For this review, take the finished solid that the model builds, in its own axes (mm). A direction names the side the tool comes from. Coordinates: 2 decimals unless noted, no trailing zeros. Write each loop counter-clockwise with the first axis right and the second up, starting at its lowest first coordinate (ties: lowest second). Pieces come first, ordered by that corner, then holes. Notation, with made-up numbers: M -36,41.25 L -18,41.25 A20 ccw -18,48.25 Z; hole C 15.5,16.5 d4. An arc over 180 degrees is marked long. Return JSON: item names as keys, results as strings.
```python
from build123d import *

# Parameters (mm, degrees)
F0_R     = 25.4
F1_DEPTH = 228.6
F0_W     = 1422.4
F0_H     = 254
F2_DEPTH = 101.6
F3_DEPTH = 635
F4_W     = 457.2
F4_H     = 177.8
F5_DEPTH = 76.2


with BuildPart() as f1:
    # F0 (on Top) → F1 (new body)
    with BuildSketch(Plane.XY):
        with BuildLine():
            Line((0, 508), (0, 254))
            Line((0, 254), (1422.4, 254))
            Line((1422.4, 254), (1422.4, 508))
            add(Edge.make_bspline(
                [(0, 508), (241.551548, 567.851314), (711.2, 651.348686), (1180.848452, 567.851314), (1422.4, 508)],
                knots=[0, 0, 0, 0, 718.42049, 1436.840979, 1436.840979, 1436.840979, 1436.840979], degree=3))
        make_face()
        with Locations((546.1, 558.8)):
            Circle(F0_R, mode=Mode.SUBTRACT)
        with Locations((876.3, 558.8)):
            Circle(F0_R, mode=Mode.SUBTRACT)
        with Locations((546.1, 558.8)):
            Circle(F0_R)
        with Locations((876.3, 558.8)):
            Circle(F0_R)
    extrude(amount=F1_DEPTH)

    # F0 (on Top) → F2 (join)
    with BuildSketch(Plane.XY):
        with Locations((711.2, 127)):
            Rectangle(F0_W, F0_H)
        with Locations((88.9, 76.2)):
            Circle(F0_R, mode=Mode.SUBTRACT)
        with Locations((1333.5, 76.2)):
            Circle(F0_R, mode=Mode.SUBTRACT)
        with Locations((88.9, 76.2)):
            Circle(F0_R)
        with Locations((1333.5, 76.2)):
            Circle(F0_R)
    extrude(amount=F2_DEPTH)

    # F0 (on Top) → F3 (join)
    with BuildSketch(Plane.XY):
        with Locations((876.3, 558.8)):
            Circle(F0_R)
        with Locations((546.1, 558.8)):
            Circle(F0_R)
        with Locations((1333.5, 76.2)):
            Circle(F0_R)
        with Locations((88.9, 76.2)):
            Circle(F0_R)
    extrude(amount=-F3_DEPTH)

    # F4 (on face) → F5 (join)
    with BuildSketch(Plane(origin=(0, 0, -635), x_dir=(1, 0, 0), z_dir=(0, 0, -1))):
        with Locations((711.2, -520.7)):
            Rectangle(F4_W, F4_H)
    extrude(amount=-F5_DEPTH)


solid = f1.part
```
1. Draft analysis for pull direction X (two halves, no side actions). For faces 4 (the face through (1308.125, 77.317, -313.055)), 5 (the face through (701, 129, 101.6)), 6 (the face through (1422.4, 307, 87)), state which applies: +X half, -X half, draft (parallel to the pull), parting line (faces both ways), or undercut.
Checks:
{"face 4": "undercut", "face 5": "draft", "face 6": "+X half"}
2. We need section A-A (z = -462.5). State the section outline as (x, y) points, plus the area to 3 significant figures.
Checks:
{"outline": "C 88.9,76.2 d50.8; C 546.1,558.8 d50.8; C 876.3,558.8 d50.8; C 1333.5,76.2 d50.8", "area": "8,110 mm2"}
3. We need section B-B (y = 76.2). State the section outline as (x, z) points.
Checks:
{"outline": "M 0,0 L 63.5,0 L 63.5,-635 L 114.3,-635 L 114.3,0 L 1308.1,0 L 1308.1,-635 L 1358.9,-635 L 1358.9,0 L 1422.4,0 L 1422.4,101.6 L 0,101.6 Z"}
4. For faces 1 (the face through (856.143, 543.344, -275.488)), 2 (the face through (708, 431.8, -597)), 3 (the face through (939.8, 522, -597)), list the 3-axis set-ups (+Z, -Z, +X, -X, +Y, -Y) from which the entire face can be reached by the end or side of a thin tool; tool diameter is ignored.
Checks:
{"face 1": "none", "face 2": "-Z, +X, -X, -Y", "face 3": "-Z, +X, +Y, -Y"}
5. Clearance check with flat-ended pins moving along their axes: pin 1 Ø2 at (x, y) = (680.5, 159.5) entering from -Z; pin 2 Ø23 at (x, z) = (678.5, -601.5) entering from -Y; pin 3 Ø3 at (x, y) = (839, 70.5) entering from +Z. State where each tip first meets the part, or that it passes through.
Checks:
{"pin 1": "z = 0", "pin 2": "y = 431.8", "pin 3": "z = 101.6"}
6. We need section C-C (y = 305.5). State the section outline as (x, z) points.
Checks:
{"outline": "M 0,0 L 1422.4,0 L 1422.4,228.6 L 0,228.6 Z"}
7. Wall thickness on L1, parallel to Z at x = 496.5, y = 498; L2, parallel to Z at x = 1269.5, y = 420; L3, parallel to Z at x = 207, y = 203: over which ranges is each line inside the solid? List them lowest first. Write a range as from..to.
Checks:
{"L1": "-635..-558.8, 0..228.6", "L2": "0..228.6", "L3": "0..101.6"}
8. We need section D-D (y = 145.5). State the section outline as (x, z) points, plus the area to 3 significant figures.
Checks:
{"outline": "M 0,0 L 1422.4,0 L 1422.4,101.6 L 0,101.6 Z", "area": "145,000 mm2"}
